Here's the drawing with two shaded views (mm, measured from the low corner). I have some questions. Coordinates: 2 decimals unless noted, no trailing zeros. Write each loop counter-clockwise with the first axis right and the second up, starting at its lowest first coordinate (ties: lowest second). Pieces come first, ordered by that corner, then holes. Notation, with made-up numbers: (10, 37.25) -> (58, 37.25) arc R13 cw to (58, 53.25) -> close; hole circle Ø9 at (16, 51). An arc over 180 degrees is marked (long way). Put each result on its own line as item: value.
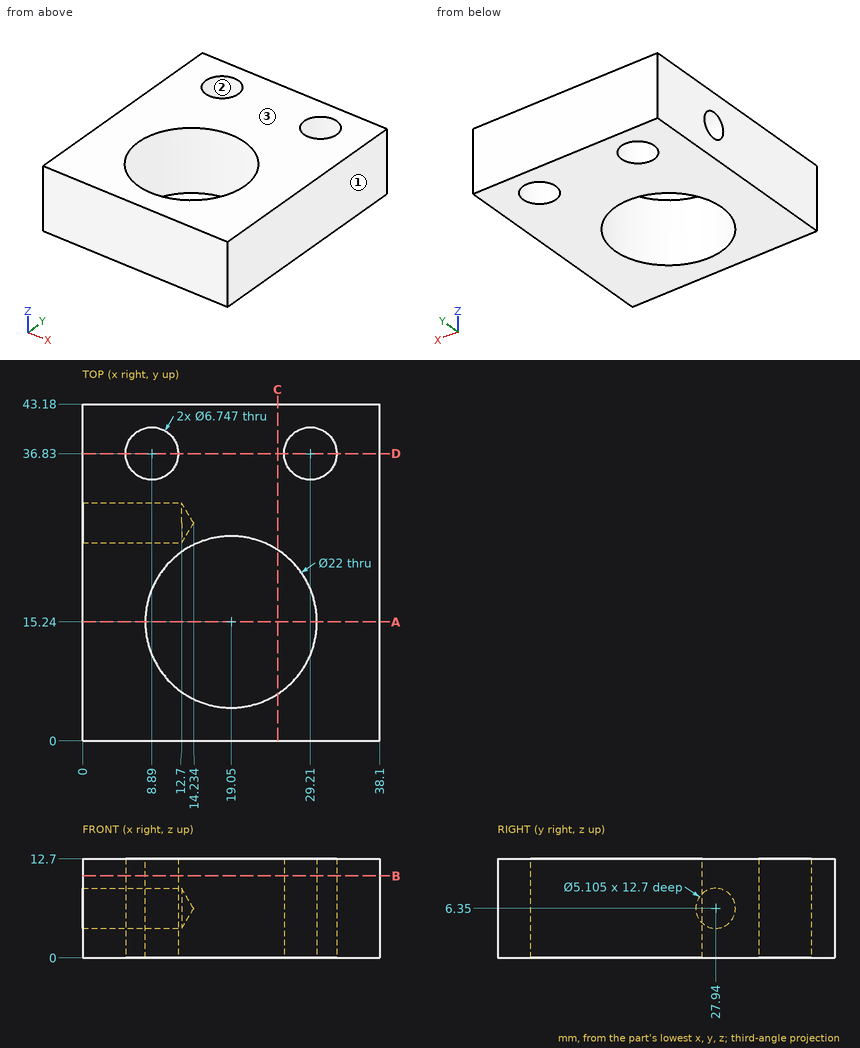
Item 1: Imagine slicing it at A-A on y = 15.24. Write out the boundary of the cut face in (x, z).
Output:
outline: (0, 0) -> (8.05, 0) -> (8.05, 12.7) -> (0, 12.7) -> close; (30.05, 0) -> (38.1, 0) -> (38.1, 12.7) -> (30.05, 12.7) -> close
Item 2: For P1, Ø17.5, axis at x = 19.05, y = 15.24, coming from the -Z side; P2, Ø11, axis at x = 29.21, y = 36.83, coming from the +Z side, each with a flat end and sliding along its axis, tell me the tip position at first contact or that it passes through.
Output:
P1: passes through
P2: stops at z = 12.7
Item 3: Imagine slicing it at B-B on z = 10.5. Write out the boundary of the cut face in (x, y), then the cut area to 3 significant figures.
Output:
outline: (0, 0) -> (38.1, 0) -> (38.1, 43.18) -> (0, 43.18) -> close; hole circle Ø6.75 at (8.89, 36.83); hole circle Ø22 at (19.05, 15.24); hole circle Ø6.75 at (29.21, 36.83)
area: 1,190 mm²
Item 4: Please list where these lines run through material, in increasing order: line 1 along Z through (x, y) = (6.5, 27.94); line 2 along Y through (x, z) = (28, 12) (1 decimal); line 3 along Y through (x, z) = (6.25, 6.35) (1 decimal). Write a range as from..to.
Output:
line 1: z = 0..3.8, 8.9..12.7
line 2: y = 0..8.8, 21.6..33.7, 40..43.2
line 3: y = 0..25.4, 30.5..34.7, 38.9..43.2
Item 5: Imagine slicing it at C-C on x = 25. Write out the boundary of the cut face in (y, z), then the cut area to 3 significant figures.
Output:
outline: (0, 0) -> (5.99, 0) -> (5.99, 12.7) -> (0, 12.7) -> close; (24.49, 0) -> (43.18, 0) -> (43.18, 12.7) -> (24.49, 12.7) -> close
area: 313 mm²
Item 6: If we mould it in two halves opening along X, with no side actions, what happens to the marked faces 1, 2 and 3? For each: released by +X, released by -X, zero draft, split by the parting line, or undercut.
Output:
face 1: released by +X
face 2: undercut
face 3: zero draft
Item 7: Imagine slicing it at D-D on y = 36.83. Write out the boundary of the cut face in (x, z).
Output:
outline: (0, 0) -> (5.52, 0) -> (5.52, 12.7) -> (0, 12.7) -> close; (12.26, 0) -> (25.84, 0) -> (25.84, 12.7) -> (12.26, 12.7) -> close; (32.58, 0) -> (38.1, 0) -> (38.1, 12.7) -> (32.58, 12.7) -> close
